Geometry: see drawing. Coordinates: mm, zero at the bounding-box minimum. A direction names the side the tool comes from. Round coordinates to 2 decimals unless told otherwise and drop trailing zeros. Order: outer loops, then holes, each group sorted by start corner. A loop starts at its lowest first (then second) coordinate and runs counter-clockwise, first axis right, second up. Notation, with made-up numbers: (7.5, 73) - (41.5, 73) arc R11 cw to (41.5, 83) - close; hole circle Ø10 at (-8, 75). An arc over 180 degrees is marked (long way). Put each result on its own line as item: value. Start each with the question number.
1) Line query: probe 1 along X at (y, z) = (13.75, 39); probe 2 along Y at (x, z) = (85, 2); probe 3 along X at (y, z) = (28.5, 9.5). Output: solid intervals per line, ascending. Write a range as [from, to].
2) Contact query for flat-ended pins moving along their axis: P1, Ø10, axis at x = 113, y = 18, coming from the +Z side; P2, Ø9, axis at x = 72, y = 13, coming from the +Z side; P3, Ø4, axis at x = 24, y = 7.5, coming from the +Z side; P4, Ø2.5, axis at x = 85, y = 15, coming from the -Z side. Output: stop coordinate, or through.
3) Section D-D on y = 15. State how many separate pieces and enclosed holes the cut face has, then the cut area to 3 significant figures.
4) Mould query, pull axis Z, two halves, no side actions, for the marked faces 4, 5 and 6. Classes: +Z half, -Z half, draft (parallel to the pull), parting line (faces both ways), or undercut.
5) Section B-B on x = 85. Output: boundary loops of the cut face in (y, z).
6) Section A-A on z = 45. Output: boundary loops of the cut face in (x, y).
7) Access query for the marked faces 1, 2 and 3. Directions: +Z, -Z, +X, -X, +Y, -Y. A direction counts if a zero-diameter tool reaches every point of the face in a straight line with its end or side. Return the directions, or none.
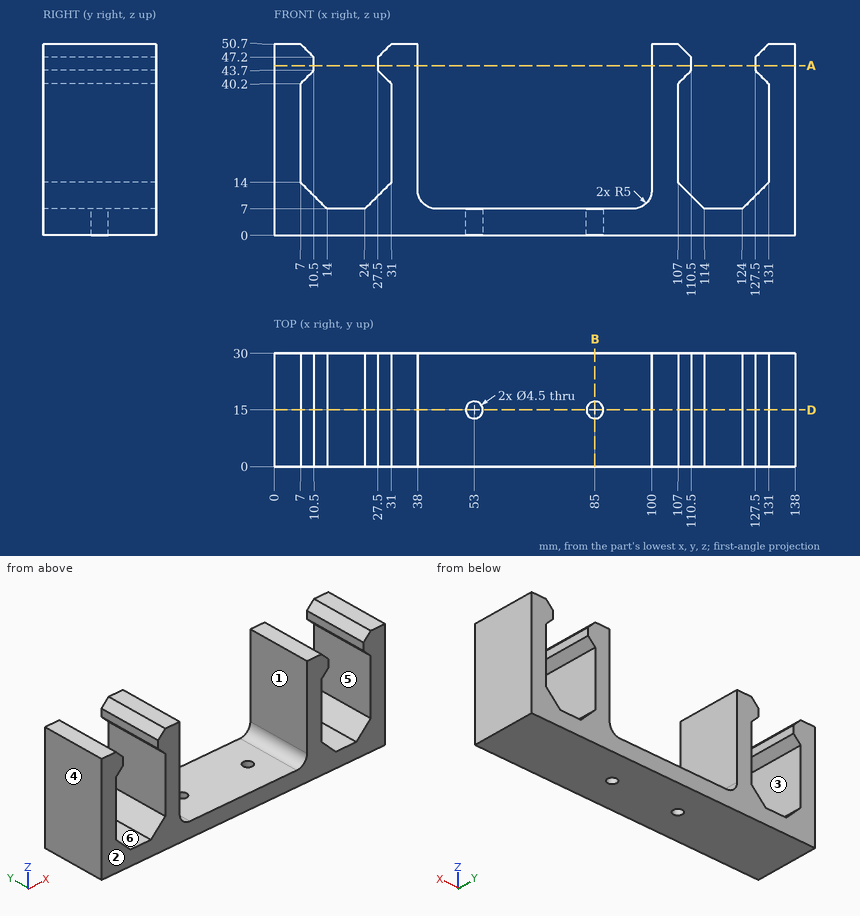
Answer sheet:
1. probe 1: [0, 7], [31, 38], [100, 107], [131, 138]
1. probe 2: [0, 12.75], [17.25, 30]
1. probe 3: [0, 11.5], [26.5, 38.67], [99.33, 111.5], [126.5, 138]
2. P1: z = 49.7
2. P2: z = 7
2. P3: z = 9
2. P4: through
3. separate pieces: 3
3. enclosed holes: 0
3. area: 2,330 mm^2
4. face 4: draft
4. face 5: undercut
4. face 6: +Z half
5. outline: (0, 0) - (12.75, 0) - (12.75, 7) - (0, 7) - close; (17.25, 0) - (30, 0) - (30, 7) - (17.25, 7) - close
6. outline: (0, 0) - (10.5, 0) - (10.5, 30) - (0, 30) - close; (27.5, 0) - (38, 0) - (38, 30) - (27.5, 30) - close; (100, 0) - (110.5, 0) - (110.5, 30) - (100, 30) - close; (127.5, 0) - (138, 0) - (138, 30) - (127.5, 30) - close
7. face 1: +Z, +Y, -Y
7. face 2: +Z, -Z, +X, -X, -Y
7. face 3: +Y, -Y
